Could you check a few things on this model? Use its own coordinates, in mm. Face numbers are marked on the shaded views. A direction names the side the tool comes from. Give positions to 0.01 mm unless a question says otherwise; leave off trailing zeros. Order: outer loops, then holes, each group sorted by start corner. A loop starts at its lowest first (then second) coordinate and runs counter-clockwise, first axis right, second up. Notation, with made-up numbers: (0.5, -17.5) -> (24.5, -17.5) arc R20 ccw to (24.5, 1.5) -> close; hole circle Ø10 at (8, -35). An arc over 180 degrees is marked (long way). One line per item, written item: value.
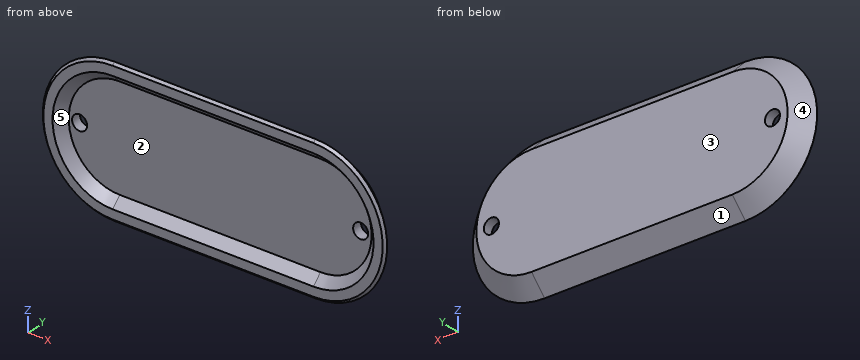
```python
from build123d import *
from OCP.BRepFilletAPI import BRepFilletAPI_MakeChamfer

# Parameters (mm, degrees)
BOSS_EXTRU_1_DEPTH      = 3.8
BOSS_EXTRU_1_TAPER      = 45
COQUE2_DEPTH            = 1.8
COQUE2_DRAFT            = 45
CHANFREIN1_SIZE         = 1
CHANFREIN1_SIZE2        = 0.707106781
ENL_V_MAT_EXTRU_1_REACH = 39.355
ESQUISSE2_R             = 1.5


# Read off the part's stored shape, not the designer's step: Coque2
with BuildPart() as part:
    # Esquisse1 → Boss.-Extru.1 (new body)
    with BuildSketch(Plane(origin=(0, 0, 0), x_dir=(1, 0, 0), z_dir=(0, 1, 0))):
        with BuildLine():
            ThreePointArc((-20, 14.8), (-34.8, 0), (-20, -14.8))
            Line((-20, -14.8), (20, -14.8))
            ThreePointArc((20, -14.8), (34.8, 0), (20, 14.8))
            Line((20, 14.8), (-20, 14.8))
        make_face()
    extrude(amount=BOSS_EXTRU_1_DEPTH, taper=BOSS_EXTRU_1_TAPER)


with BuildPart() as coque2_tool:
    # Coque2 outline → Coque2 (with draft: the straight prism first)
    with BuildSketch(Plane(origin=(0, 1.8, 0), x_dir=(1, 0, 0), z_dir=(0, 1, 0))):
        with BuildLine():
            Line((-20, -10.171572875), (20, -10.171572875))
            ThreePointArc((20, -10.171572875), (30.171572875, 0), (20, 10.171572875))
            Line((20, 10.171572875), (-20, 10.171572875))
            ThreePointArc((-20, 10.171572875), (-30.171572875, 0), (-20, -10.171572875))
        make_face()
    extrude(amount=-COQUE2_DEPTH)
    # Coque2: the draft: its side faces are tilted about the plane it starts from
    coque2_sides = [coque2_tool.faces().sort_by_distance(p)[0] for p in [
        (0, 0.9, 10.171572875),
        (30.171572875, 0.9, 0),
        (0, 0.9, -10.171572875),
        (-30.171572875, 0.9, 0),
    ]]
    draft(coque2_sides, Plane(origin=(0, 1.8, 0), x_dir=(1, 0, 0), z_dir=(0, 1, 0)), COQUE2_DRAFT)


with BuildPart() as part_1:
    add(part.part)

    # Coque2: cut by coque2_tool
    add(coque2_tool.part, mode=Mode.SUBTRACT)

    # Chanfrein1: one chamfer whose edges measure the first distance from different faces: ONE call of the kernel's chamfer builder (chamfer() names one face for all edges)
    chanfrein1_edges_1 = [part_1.edges().sort_by_distance(p)[0] for p in [
        (0, 0, -14.8),
        (0, 0, 14.8),
        (-34.8, 0, 0),
    ]]
    chanfrein1_side_1 = [part_1.faces().sort_by_distance(p)[0] for p in [
        (0, 0, -14.043672029),
    ]]
    chanfrein1_edges_2 = [part_1.edges().sort_by_distance(p)[0] for p in [
        (34.8, 0, 0),
    ]]
    chanfrein1_side_2 = [part_1.faces().sort_by_distance(p)[0] for p in [
        (32.9, 1.9, 0),
    ]]
    chanfrein1 = BRepFilletAPI_MakeChamfer(part_1.part.solid().wrapped)
    for e in chanfrein1_edges_1:
        chanfrein1.Add(CHANFREIN1_SIZE, CHANFREIN1_SIZE2, e.wrapped, chanfrein1_side_1[0].wrapped)  # the first distance lies on this face
    for e in chanfrein1_edges_2:
        chanfrein1.Add(CHANFREIN1_SIZE, CHANFREIN1_SIZE2, e.wrapped, chanfrein1_side_2[0].wrapped)  # the first distance lies on this face
    add(Compound.cast(chanfrein1.Shape()), mode=Mode.REPLACE)

    # Esquisse2 → Enlèv. mat.-Extru.1 (cut, up to next)
    with BuildSketch(Plane(origin=(0, 3.8, 0), x_dir=(1, 0, 0), z_dir=(0, 1, 0)), mode=Mode.PRIVATE) as enl_v_mat_extru_1_sk1:
        with Locations(Location((-28, 0, 0), (0, 0, 270))):
            Circle(ESQUISSE2_R)
    enl_v_mat_extru_1_tool1 = extrude(enl_v_mat_extru_1_sk1.sketch, amount=-ENL_V_MAT_EXTRU_1_REACH, mode=Mode.PRIVATE) & part_1.part
    # Esquisse2 → Enlèv. mat.-Extru.1 (cut, up to next)
    with BuildSketch(Plane(origin=(0, 3.8, 0), x_dir=(1, 0, 0), z_dir=(0, 1, 0)), mode=Mode.PRIVATE) as enl_v_mat_extru_1_sk2:
        with Locations(Location((28, 0, 0), (0, 0, 270))):
            Circle(ESQUISSE2_R)
    enl_v_mat_extru_1_tool2 = extrude(enl_v_mat_extru_1_sk2.sketch, amount=-ENL_V_MAT_EXTRU_1_REACH, mode=Mode.PRIVATE) & part_1.part
    add(enl_v_mat_extru_1_tool1.solids().sort_by_distance((-28, 3.8, 0))[0], mode=Mode.SUBTRACT)
    add(enl_v_mat_extru_1_tool2.solids().sort_by_distance((28, 3.8, 0))[0], mode=Mode.SUBTRACT)


solid = part_1.part
```
1) Suppose I cut it at A-A, the plane y = 3.05. Write out the boundary of the cut face in (x, z), then the cut area to 3 significant figures.
Answer below:
outline: (-20, -11.75) -> (20, -11.75) arc R11.75 ccw to (20, 11.75) -> (-20, 11.75) arc R11.75 ccw to start; hole circle Ø3 at (-28, 0); hole circle Ø3 at (28, 0)
area: 1,360 mm2
2) We'd pull the mould along X, two halves only. Please class the marked faces 3, 4 and 5: +X half, -X half, draft (parallel to the pull), parting line (faces both ways), or undercut.
Answer below:
face 3: draft
face 4: -X half
face 5: undercut
3) For P1, Ø3, axis at x = 20.5, z = -2.5, coming from the -Y side; P2, Ø1.5, axis at x = 21.5, y = 2, coming from the -Z side, each with a flat end and sliding along its axis, tell me the tip position at first contact or that it passes through.
Answer below:
P1: stops at y = 1.8
P2: stops at z = -13.47
4) Suppose I cut it at C-C, the plane z = -0.25. State how many separate pieces and enclosed holes the cut face has, then the cut area to 3 significant figures.
Answer below:
separate pieces: 3
enclosed holes: 0
area: 126 mm2
5) For the marked faces 1 and 2, which set-ups out of +Z, -Z, +X, -X, +Y, -Y let a thin tool reach every point of the face, with its end or its side?
Answer below:
face 1: -Z, +X, -X, +Y
face 2: -Y
6) Suppose I cut it at B-B, the plane x = 7.5. Write out the boundary of the cut face in (y, z), then the cut area to 3 significant figures.
Answer below:
outline: (0, -13.8) -> (0.5, -14.3) -> (3.8, -11) -> (3.8, 11) -> (0.5, 14.3) -> (0, 13.8) -> (0, 11.97) -> (1.8, 10.17) -> (1.8, -10.17) -> (0, -11.97) -> close
area: 57.7 mm2
7) If I drill on line 1 along X through (y, z) = (3.2, 0); line 2 along X through (y, z) = (3.2, 0.5); line 3 along Y through (x, z) = (10.5, -3.25), over which ranges is the centre line in solid material (lowest first)?
Answer below:
line 1: x = -31.6 to -29.5, -26.5 to 26.5, 29.5 to 31.6
line 2: x = -31.59 to -29.41, -26.59 to 26.59, 29.41 to 31.59
line 3: y = 1.8 to 3.8
